```python
from build123d import *

# Parameters (mm, degrees)
BOSS_EXTRUDE1_DEPTH     = 6.35
FILLET1_R               = 12.7
CUT_EXTRUDE1_DEPTH      = 44.067795393
CUT_EXTRUDE1_DEPTH_BACK = 44.067795393
SKETCH2_W               = 6.35
SKETCH2_H               = 50.113024572


with BuildPart() as part:
    # Sketch1 → Boss-Extrude1 (new body)
    with BuildSketch(Plane.XY):
        Polygon((-9.525, -31.75), (9.525, -31.75), (9.525, -38.1), (19.05, -38.1), (19.05, -31.75), (19.05, 19.05), (0, 25.4), (-19.05, 19.05), (-19.05, -31.75), (-19.05, -38.1), (-9.525, -38.1), align=None)
    extrude(amount=BOSS_EXTRUDE1_DEPTH)

    # Fillet1
    fillet1_edges = [part.edges().sort_by_distance(p)[0] for p in [
        (-19.05, 19.05, 3.175),
        (0, 25.4, 3.175),
        (19.05, 19.05, 3.175),
    ]]
    fillet(fillet1_edges, radius=FILLET1_R)

    # Sketch2 → Cut-Extrude1 (cut, two sides: drawn at the far end of the back side and taken through both)
    with BuildSketch(Plane.XY.offset(6.35).offset(-CUT_EXTRUDE1_DEPTH_BACK)):
        with Locations((0, -6.693487714)):
            Rectangle(SKETCH2_W, SKETCH2_H)
    extrude(amount=CUT_EXTRUDE1_DEPTH + CUT_EXTRUDE1_DEPTH_BACK, mode=Mode.SUBTRACT)


solid = part.part
```
Could you check a few things on this model? Use its own coordinates, in mm. A direction names the side the tool comes from. Give positions to 0.01 mm unless a question says otherwise; leave off trailing zeros. Write each loop counter-clockwise with the first axis right and the second up, starting at its lowest first coordinate (ties: lowest second). Pieces come first, ordered by that corner, then holes. Notation, with made-up numbers: (3.5, 7.5) - (10.5, 7.5) arc R23 cw to (10.5, 23.5) - close; hole circle Ø5 at (54.25, 61). An arc over 180 degrees is marked (long way). One line per item, written item: value. Start each with the question number.
Item 1: If we mould it in two halves opening along X, with no side actions, what happens to faces 3 (the face through (19.05, -14, 3)), 4 (the face through (14, -38.1, 3)), 5 (the face through (3.175, -7, 3)), 6 (the face through (6, -31.75, 3))? For each: +X half, -X half, draft (parallel to the pull), parting line (faces both ways), or undercut.
Item 2: Imagine slicing it at D-D, the plane x = 0. List the corners of the cut face in (y, z) for me, and give its area (3 significant figures).
Item 3: Imagine slicing it at A-A, the plane y = -25.5. List the corners of the cut face in (x, z) for me (3 decimals), and give its area (3 significant figures).
Item 4: I'm going to push flat-ended pins straight in: pin 1 (3 mm diameter, centred on x = -5.5, z = 4.5, fed in from -Y); pin 2 (1.5 mm diameter, centred on x = -1, z = 3, fed in from +Y); pin 3 (1 mm diameter, centred on x = 14, z = 5, fed in from +Y). Where does each tip first touch, or does it pass through?
Item 5: Imagine slicing it at C-C, the plane x = -6. List the corners of the cut face in (y, z) for me.
Item 6: Imagine slicing it at B-B, the plane z = 0.75. List the corners of the cut face in (x, y) for me (3 decimals).
Item 7: Which directions (+Z, -Z, +X, -X, +Y, -Y) give clear straight access to the entire face, cutting with the end or side of a thin tool? Please do faces 1 (the face through (-16.59, 17.41, 3.22)), 2 (the face through (-3.175, -7, 3)).
Item 8: Please list where these lines run through material, in increasing order: line 1 (X direction, y = -8, z = 1) (3 decimals); line 2 (Y direction, x = 0, z = 1.5). Write a range as from..to.
Geometry says:
1. face 3: +X half
1. face 4: draft
1. face 5: undercut
1. face 6: undercut
2. outline: (18.36, 0) - (24.71, 0) - (24.71, 6.35) - (18.36, 6.35) - close
2. area: 40.3 mm^2
3. outline: (-19.05, 0) - (-3.175, 0) - (-3.175, 6.35) - (-19.05, 6.35) - close; (3.175, 0) - (19.05, 0) - (19.05, 6.35) - (3.175, 6.35) - close
3. area: 202 mm^2
4. pin 1: y = -31.75
4. pin 2: y = 24.71
4. pin 3: y = 20.39
5. outline: (-31.75, 0) - (23.4, 0) - (23.4, 6.35) - (-31.75, 6.35) - close
6. outline: (-19.05, -38.1) - (-9.525, -38.1) - (-9.525, -31.75) - (-3.175, -31.75) - (-3.175, 18.363) - (3.175, 18.363) - (3.175, -31.75) - (9.525, -31.75) - (9.525, -38.1) - (19.05, -38.1) - (19.05, 9.896) arc R12.7 ccw to (10.366, 21.945) - (4.016, 24.061) arc R12.7 ccw to (-4.016, 24.061) - (-10.366, 21.945) arc R12.7 ccw to (-19.05, 9.896) - close
7. face 1: +Z, -Z, -X, +Y
7. face 2: +Z, -Z, -Y
8. line 1: -19.05..-3.175, 3.175..19.05
8. line 2: 18.36..24.71
